The listing builds one solid part. Answer for the finished solid, in the listing's coordinates (mm). A direction names the side the tool comes from. Round coordinates to 2 decimals unless told otherwise and drop trailing zeros. Write each loop counter-clockwise with the first axis right and the second up, starting at its lowest first coordinate (ties: lowest second). Pieces come first, ordered by that corner, then holes. Notation, with made-up numbers: (-37.75, 61) - (-29.75, 61) arc R8 ccw to (-29.75, 65) - close; hole circle Ø1 at (35.25, 38). An arc over 180 degrees is marked (long way). Return JSON: item names as keys, results as strings. Group by question number.
(1) Section C-C, the plane z = 0 is taken. Write down the section's boundary in (x, y) (1 decimal), then the cut area to 3 significant figures.
(2) Which of the six approach directions +Z, -Z, +X, -X, +Y, -Y give full straight-line access (tool end or side, diameter ignored) to faces 1 (the cylindrical face through (18.421, 37.126, 0.909)), 2 (the flat face through (1.6, 22.4, -19.1))?
(3) Find the intervals of material crossed by line 1 along Z through (x, y) = (15, -9.5); line 2 along Y through (x, z) = (22, 0) (3 decimals); line 3 along Y through (x, z) = (3, -2.5) (3 decimals), in increasing order. Write a range as [from, to].
(4) Each of these flat-tipped pins is pushed along its axis until it touches: pin 1 (6 mm diameter, centred on x = 10.5, y = 32.5, fed in from +Z); pin 2 (8.5 mm diameter, centred on x = 15, z = -29.39, fed in from +Y); pin 3 (2 mm diameter, centred on x = 11, z = 24, fed in from +Y) (3 decimals). Where does it stop, or does it pass through?
(5) Section D-D, the plane x = 25 is taken. Write down the section's boundary in (y, z) (1 decimal).
(6) Section B-B, the plane y = 3.5 is taken. Write down the section's boundary in (x, z) (3 decimals), then the cut area to 3 significant figures.
(7) Determine the mould class of faces 3 (the flat face through (0.8, 15.09, -26.09)), 4 (the flat face through (6.604, 27, 10)), 5 (the cylindrical face through (4.06, 15.89, -0.63)), 6 (the flat face through (1.61, -0.583, -36.535)) for opening direction Z: +Z half, -Z half, draft (parallel to the pull), parting line (faces both ways), or undercut.
(8) Section A-A, the plane x = 15 is taken. Write down the section's boundary in (y, z) (1 decimal).
Autodesk Inventor part; units mm, degrees
ref_plane "YZ Plane" through (0, 0, 0) normal (1, 0, 0) x (0, 1, 0)
ref_plane "XZ Plane" through (0, 0, 0) normal (0, 1, 0) x (-1, 0, 0)
ref_plane "XY Plane" through (0, 0, 0) normal (0, 0, 1) x (1, 0, 0)
sketch "Sketch1" plane through (0, 0, 0) normal (1, 0, 0) x (0, 1, 0)
  line L0 (-15.875, 38.1) -> (15.875, 38.1)
  line L1 (15.875, -38.1) -> (-15.875, -38.1)
  line L2 (-15.875, -38.1) -> (-15.875, 38.1)
  line L3 (-15.875, 38.1) -> (15.875, -38.1) construction
  line L4 (15.875, 38.1) -> (-15.875, -38.1) construction
  circle A0 centre (30.2006, 0) radius 14.3256
  line L5 (29.6902, 20.6693) -> (15.875, 20.3282)
  line L6 (30.2006, -20.6756) -> (15.875, -20.6756)
  arc A1 (30.2006, -20.6756) -> (29.6902, 20.6693) centre (30.2006, 0) ccw
  line L7 (15.875, 38.1) -> (15.875, 20.3282)
  line L8 (15.875, -20.6756) -> (15.875, -38.1)
  point P0 (0, 0)
  point P1 (0, 0)
  point P2 (0, 0)
  dimension "d0" = 31.75
  dimension "d2" = 28.6512
  dimension "d4" = 6.35
  dimension "d5" = 1.414
  dimension "d24" = 76.2
extrude "Extrusion1" add sketch "Sketch1" along normal blind 30
sketch "Sketch2" plane through (30, 0, 0) normal (1, 0, 0) x (0, 0, -1)
  circle A0 centre (0, 30.2006) radius 14.3256
  arc A1 (20.6756, 30.2006) -> (-20.6693, 29.6902) centre (0, 30.2006) ccw
  circle A2 centre (0, 30.2006) radius 6.985
  circle A3 centre (0, 30.2006) radius 14.3256
  point P0 (0, 0)
  dimension "d8" = 13.97
extrude "Extrusion2" add sketch "Sketch2" against normal blind 23.396
sketch "Sketch3" plane through (0, 15.875, -20.6756) normal (0, 1, 0) x (1, 0, 0)
  line L0 (30, 0) -> (0, 17.4244)
  line L1 (30, -41.0038) -> (30, -58.7756)
  line L2 (0, -41.0038) -> (30, -41.0038)
  line L3 (30, -58.7756) -> (0, -41.0038)
  point P0 (0, -20.6756)
  point P1 (15, -49.8897)
  point P2 (15, 8.7122)
hole "Hole1" at (15, 15.875, 29.2141) at (15, 15.875, -29.3878) direction (0, -1, 0) diameter 6.604 end through all countersink diameter 12.5984 countersink angle 90
chamfer "Chamfer1" distance 3.175 angle 45 12 edges at (0, 0, 38.1) (30, 0, 38.1) (0, 0, -38.1) (30, 0, -38.1) (0, 50.8746, 0.2552) (0, 23.0378, -20.6756) (0, 22.7826, 20.4987) (30, 50.8746, 0.2552) (30, 22.7826, 20.4987) (30, 23.0378, -20.6756) (30, 30.2006, 6.985) (6.604, 30.2006, 6.985)
chamfer "Chamfer2" distance 1.5875 angle 45 11 edges at (0, 15.875, -27.8003) (15, 15.875, -38.1) (30, 15.875, -27.8003) (30, 15.875, 27.6266) (28.4125, 15.875, 36.5125) (15, 15.875, 38.1) (1.5875, 15.875, 36.5125) (0, 15.875, 27.6266) (1.5875, 15.875, -36.5125) (28.4125, 15.875, -36.5125) (0, 15.875, 0)
properties part number "2316_Pillow Block_V1"
Working result:
{
 "1": {"outline": "(0, -15.9) - (30, -15.9) - (30, 20) - (26.8, 23.2) - (9.8, 23.2) - (6.6, 20) - (6.6, 15.9) - (1.6, 15.9) - (0, 14.3) - close; (0, 46.1) - (1.6, 44.5) - (6.6, 44.5) - (6.6, 40.4) - (9.8, 37.2) - (26.8, 37.2) - (30, 40.4) - (30, 47.7) - (26.8, 50.9) - (3.2, 50.9) - (0, 47.7) - close", "area": "1,450 mm^2"},
 "2": {"face 1": "+X, -X", "face 2": "-Z, -X, +Y"},
 "3": {"line 1": "z = [-38.1, -32.69], [-26.09, 25.91], [32.52, 38.1]", "line 2": "y = [-15.875, 23.216], [37.186, 50.876]", "line 3": "y = [-15.875, 16.095], [44.306, 50.548]"},
 "4": {"pin 1": "stops at z = 20.68", "pin 2": "stops at y = 13.83", "pin 3": "stops at y = 15.875"},
 "5": {"outline": "(-15.9, -38.1) - (14.3, -38.1) - (15.9, -36.5) - (15.9, -20.7) - (30.2, -20.7) arc R20.7 ccw (long way) to (29.7, 20.7) - (15.9, 20.3) - (15.9, 36.5) - (14.3, 38.1) - (-15.9, 38.1) - close; hole circle Ø14 at (30.2, 0)"},
 "6": {"outline": "(0, -34.925) - (3.175, -38.1) - (26.825, -38.1) - (30, -34.925) - (30, 34.925) - (26.825, 38.1) - (3.175, 38.1) - (0, 34.925) - close; hole circle Ø6.604 at (15, -29.388); hole circle Ø6.604 at (15, 29.214)", "area": "2,200 mm^2"},
 "7": {"face 3": "draft", "face 4": "undercut", "face 5": "undercut", "face 6": "-Z half"},
 "8": {"outline": "(-15.9, -38.1) - (14.3, -38.1) - (15.9, -36.5) - (15.9, -35.7) - (12.9, -32.7) - (-15.9, -32.7) - close; (-15.9, -26.1) - (12.9, -26.1) - (15.9, -23.1) - (15.9, -20.7) - (30.2, -20.7) arc R20.7 ccw (long way) to (29.7, 20.7) - (15.9, 20.3) - (15.9, 22.9) - (12.9, 25.9) - (-15.9, 25.9) - close; (-15.9, 32.5) - (12.9, 32.5) - (15.9, 35.5) - (15.9, 36.5) - (14.3, 38.1) - (-15.9, 38.1) - close; hole circle Ø14 at (30.2, 0)"}
}
